Can you work these out from the model? Positions are in its coordinate system, mm. A direction names the side the tool comes from. Round coordinates to 2 decimals unless told otherwise and drop trailing zeros. Loops run counter-clockwise (first coordinate to the right, second up) from the corner with the lowest first, then second, coordinate; pieces in that order, holes last. Notation, with made-up numbers: M -20,6 L 27,6 A31 ccw 27,30 Z; hole C -6.5,52 d2. An arc over 180 degrees is marked long. Return JSON: item names as keys, results as strings.
```python
from build123d import *

# Parameters (mm, degrees)
F0_W     = 111.5
F0_H     = 70
F1_DEPTH = 17
F2_W     = 108
F2_H     = 66
F3_DEPTH = 15
F4_W     = 104.5
F4_H     = 63
F5_DEPTH = 17.001


# Not quite as in the source:
# - a feature of the source that left no trace in its solid (it failed there, or was rolled back) is left out


with BuildPart() as f1:
    # F0 (on Top) → F1 (new body)
    with BuildSketch(Plane.XY):
        with Locations((55.75, 35)):
            Rectangle(F0_W, F0_H)
    extrude(amount=F1_DEPTH)

    # F2 (on face) → F3 (cut)
    with BuildSketch(Plane.XY.offset(17)):
        with Locations((55.75, 35)):
            Rectangle(F2_W, F2_H)
    extrude(amount=-F3_DEPTH, mode=Mode.SUBTRACT)

    # F4 (on face) → F5 (cut, through all)
    with BuildSketch(Plane(origin=(0, 0, 0), x_dir=(1, 0, 0), z_dir=(0, 0, -1))):
        with Locations((55.75, -35)):
            Rectangle(F4_W, F4_H)
    extrude(amount=-F5_DEPTH, mode=Mode.SUBTRACT)


solid = f1.part
```
Q1. Suppose I cut it at B-B, the plane x = 55.5. Please give me the cut outline in (y, z).
Results:
{"outline": "M 0,0 L 3.5,0 L 3.5,2 L 2,2 L 2,17 L 0,17 Z; M 66.5,0 L 70,0 L 70,17 L 68,17 L 68,2 L 66.5,2 Z"}
Q2. If I drill on line 1 along Y through (x, z) = (24.5, 4.75); line 2 along X through (y, z) = (59.5, 10.5); line 3 along Y through (x, z) = (11, 1.5), over which ranges is the centre line in solid material (lowest first)?
Results:
{"line 1": "y = 0 to 2, 68 to 70", "line 2": "x = 0 to 1.75, 109.75 to 111.5", "line 3": "y = 0 to 3.5, 66.5 to 70"}
Q3. Suppose I cut it at A-A, the plane y = 56.5. Please give me the cut outline in (x, z).
Results:
{"outline": "M 0,0 L 3.5,0 L 3.5,2 L 1.75,2 L 1.75,17 L 0,17 Z; M 108,0 L 111.5,0 L 111.5,17 L 109.75,17 L 109.75,2 L 108,2 Z"}
Q4. Thinking about a two-plate mould opening in Y: for faces 4 (the flat face through (39, 3, 2)), 5 (the flat face through (51, 1, 0)), 6 (the flat face through (55, 70, 8)), 7 (the flat face through (55, 0, 8)), which applies, pulls with the +Y half, pulls with the -Y half, needs draft (parallel to the pull), parting line crosses it, or undercut?
Results:
{"face 4": "undercut", "face 5": "needs draft", "face 6": "pulls with the +Y half", "face 7": "pulls with the -Y half"}
Q5. Suppose I cut it at C-C, the plane z = 11.5. Please give me the cut outline in (x, y).
Results:
{"outline": "M 0,0 L 111.5,0 L 111.5,70 L 0,70 Z; hole M 1.75,2 L 109.75,2 L 109.75,68 L 1.75,68 Z"}
Q6. On a 3-axis mill with a long thin cutter (end or side, diameter ignored), from which of +Z, -Z, +X, -X, +Y, -Y can I reach the whole of each face in a straight line? I mean faces 1 (the flat face through (55, 2, 10)), 2 (the flat face through (0, 35, 8)), 3 (the flat face through (108, 35, 1)). Say none if no direction works.
Results:
{"face 1": "+Z", "face 2": "+Z, -Z, -X, +Y, -Y", "face 3": "+Z, -Z"}
